```python
from build123d import *

# Parameters (mm, degrees)
BASES_W              = 12.5
BASES_H              = 13.35
BASE_DEPTH           = 1
SCREWACCESSS_R       = 2
SCREW_ACCESS_DEPTH   = 10.198811064
NEUTRALS_W           = 0.5
NEUTRALS_H           = 2.7
NEUTRAL_DEPTH        = 1.6
GROUNDS_W            = 2.7
GROUNDS_H            = 0.5
GROUND_DEPTH         = 1.6
EDGE_FLANGE1_START   = -6.25
EDGE_FLANGE1_DEPTH   = 12.5
EDGE_FLANGE1_2_DEPTH = 12.5


# Read off the part's stored shape, not the designer's step: Edge-Flange1
with BuildPart() as part:
    # BaseS → BASE (new body)
    with BuildSketch(Plane.XY):
        Rectangle(BASES_W, BASES_H)
    extrude(amount=-BASE_DEPTH)

    # ScrewAccessS → SCREW ACCESS (cut, through all)
    with BuildSketch(Plane.XY):
        with Locations((0, 0.875)):
            Circle(SCREWACCESSS_R)
    extrude(amount=-SCREW_ACCESS_DEPTH, mode=Mode.SUBTRACT)

    # NeutralS → NEUTRAL (cut)
    with BuildSketch(Plane.XY):
        with Locations((4.65, 0.875)):
            Rectangle(NEUTRALS_W, NEUTRALS_H)
    neutral = extrude(amount=-NEUTRAL_DEPTH, mode=Mode.SUBTRACT)

    # LINE HM: NEUTRAL across plane
    add(neutral.mirror(Plane(origin=(0, 0, 0), x_dir=(0, 0, 1), z_dir=(1, 0, 0))), mode=Mode.SUBTRACT)

    # GroundS → GROUND (cut)
    with BuildSketch(Plane.XY):
        with Locations((0, 5.425)):
            Rectangle(GROUNDS_W, GROUNDS_H)
    extrude(amount=-GROUND_DEPTH, mode=Mode.SUBTRACT)

    # Edge-Flange1 outline → Edge-Flange1 (cut)
    with BuildSketch(Plane.YZ.offset(EDGE_FLANGE1_START)):
        with BuildLine():
            Line((-6.675, 0), (-6.675, -0.049881461))
            ThreePointArc((-6.675, -0.049881461), (-6.468466602, -0.01251486), (-6.25895363, 0))
            Line((-6.25895363, 0), (-6.675, 0))
        make_face()
    extrude(amount=EDGE_FLANGE1_DEPTH, mode=Mode.SUBTRACT)

    # Edge-Flange1 2 outline → Edge-Flange1 2 (add)
    with BuildSketch(Plane.YZ.offset(EDGE_FLANGE1_START)):
        with BuildLine():
            ThreePointArc((-6.675, -0.049881461), (-6.864855726, -0.107582786), (-7.047009625, -0.186288543))
            Line((-7.047009625, -0.186288543), (-12.251294526, -2.79240029))
            Line((-12.251294526, -2.79240029), (-11.803535438, -3.686554527))
            Line((-11.803535438, -3.686554527), (-6.599250537, -1.08044278))
            ThreePointArc((-6.599250537, -1.08044278), (-6.43379143, -1.020384057), (-6.25895363, -1))
            Line((-6.25895363, -1), (-6.675, -1))
            Line((-6.675, -1), (-6.675, -0.049881461))
        make_face()
    extrude(amount=EDGE_FLANGE1_2_DEPTH)


solid = part.part
```
Design review of the part built by this model. Coordinates are the model's own, in mm. A direction names the side the tool comes from. Coordinates: 2 decimals unless noted, no trailing zeros. Order: outer loops, then holes, each group sorted by start corner. A loop starts at its lowest first (then second) coordinate and runs counter-clockwise, first axis right, second up. Notation, with made-up numbers: M 21.25,58.5 L 33.25,58.5 A23 cw 33.25,70.5 Z; hole C 54,16.5 d10. An arc over 180 degrees is marked long. Answer as a JSON object with one key per item and string values. Group by question number.
1) Add section D-D, the plane y = -7.5. Write out the cut boundary in (x, z), then the cut area to 3 significant figures.
2) Add section B-B, the plane y = 1.5. Write out the cut boundary in (x, z), then the cut area to 3 significant figures.
3) Mouldability with a two-part tool opening along Y and no side actions: class faces 4 (the flat face through (-0.09, -12.03, -3.23)), 5 (the flat face through (4.4, 0.9, -0.5)), 6 (the flat face through (-4.9, 0.9, -0.5)), 7 (the flat face through (6.25, -2.8, -0.6)) as pulls with the +Y half, pulls with the -Y half, needs draft (parallel to the pull), parting line crosses it, or undercut.
4) For pin 1 (2 mm diameter, centred on y = 4, z = -2.5, fed in from +X); pin 2 (0.5 mm diameter, centred on x = 0, z = -0.5, fed in from -Y); pin 3 (4 mm diameter, centred on x = -0.5, y = 1.5, fed in from -Z); pin 4 (1 mm diameter, centred on x = -3.5, z = -2.5, fed in from +Y), all flat-tipped, find the tip position at first contact; note any pin that passes through.
5) Add section A-A, the plane x = 0. Write out the cut boundary in (y, z) (3 decimals), then the cut area to 3 significant figures.
6) Add section C-C, the plane x = 2.5. Write out the cut boundary in (y, z) (3 decimals), then the cut area to 3 significant figures.
7) Tool access review of faces 1 (the flat face through (-1.5, -1.1, -1)), 2 (the flat face through (-4.4, 0.9, -0.5)), 3 (the flat face through (-0.1, 6.675, -0.5)): name each direction out of +Z, -Z, +X, -X, +Y, -Y from which nothing blocks a thin tool from reaching the whole face with its end or side.
8) Wall thickness on L1, parallel to Y at x = 0, z = -0.65 (3 decimals); L2, parallel to Y at x = 0, z = -0.4 (3 decimals); L3, parallel to Z at x = -1, y = -5: over which ranges is each line inside the solid? List them lowest first.
Computed values:
{
 "1": {"outline": "M -6.25,-1.53 L 6.25,-1.53 L 6.25,-0.41 L -6.25,-0.41 Z", "area": "14.0 mm^2"},
 "2": {"outline": "M -6.25,-1 L -4.9,-1 L -4.9,0 L -6.25,0 Z; M -4.4,-1 L -1.9,-1 L -1.9,0 L -4.4,0 Z; M 1.9,-1 L 4.4,-1 L 4.4,0 L 1.9,0 Z; M 4.9,-1 L 6.25,-1 L 6.25,0 L 4.9,0 Z", "area": "7.70 mm^2"},
 "3": {"face 4": "pulls with the -Y half", "face 5": "undercut", "face 6": "undercut", "face 7": "needs draft"},
 "4": {"pin 1": "passes through", "pin 2": "stops at y = -8.17", "pin 3": "stops at z = -1", "pin 4": "stops at y = -8.44"},
 "5": {"outline": "M -12.251,-2.792 L -11.804,-3.687 L -6.599,-1.08 A0.76 cw -6.259,-1 L -1.125,-1 L -1.125,0 L -6.259,0 A1.76 ccw -7.047,-0.186 Z; M 2.875,-1 L 5.175,-1 L 5.175,0 L 2.875,0 Z; M 5.675,-1 L 6.675,-1 L 6.675,0 L 5.675,0 Z", "area": "14.8 mm^2"},
 "6": {"outline": "M -12.251,-2.792 L -11.804,-3.687 L -6.599,-1.08 A0.76 cw -6.259,-1 L 6.675,-1 L 6.675,0 L -6.259,0 A1.76 ccw -7.047,-0.186 Z", "area": "19.3 mm^2"},
 "7": {"face 1": "-Z, +X, -X, +Y", "face 2": "+Z, -Z", "face 3": "+Z, -Z, +X, -X, +Y"},
 "8": {"L1": "y = -7.973 to -1.125, 2.875 to 5.175, 5.675 to 6.675", "L2": "y = -7.474 to -1.125, 2.875 to 5.175, 5.675 to 6.675", "L3": "z = -1 to 0"}
}
